Autodesk Inventor part; units mm, degrees
ref_plane "YZ Plane" through (0, 0, 0) normal (1, 0, 0) x (0, 1, 0)
ref_plane "XZ Plane" through (0, 0, 0) normal (0, 1, 0) x (-1, 0, 0)
ref_plane "XY Plane" through (0, 0, 0) normal (0, 0, 1) x (1, 0, 0)
sketch "Sketch6" plane through (0, 0, 0) normal (0, 0, 1) x (1, 0, 0)
  line L0 (20, 28) -> (24, 28)
  line L1 (24, 28) -> (24, 0)
  line L2 (24, -15) -> (20, -15)
  line L3 (20, -15) -> (20, -12)
  line L4 (17, 2) -> (20, 2)
  line L5 (20, 2) -> (20, -2) construction
  line L6 (20, -2) -> (17, -2)
  line L7 (17, -2) -> (17, 2)
  line L8 (20, -10) -> (21, -10)
  line L9 (21, -10) -> (21, -12)
  line L10 (21, -12) -> (20, -12)
  line L11 (20, -12) -> (20, -10) construction
  line L12 (20, 2) -> (20, 16)
  line L13 (20, -2) -> (20, 2) construction
  line L14 (20, -10) -> (20, -2)
  line L15 (20, -12) -> (20, -10) construction
  line L16 (0, 0) -> (0, 29.8024)
  line L17 (20, 16) -> (21, 16)
  line L18 (21, 16) -> (21, 18)
  line L19 (21, 18) -> (20, 18)
  line L20 (17, 0) -> (24, 0) construction
  line L21 (24, 0) -> (24, -15)
  line L22 (20, 18) -> (20, 28)
  line L23 (20, 16) -> (20, 18) construction
  point P0 (20, 0)
  point P1 (20, -11)
  point P2 (20.5, -10)
  dimension "d15" = 4
  dimension "d16" = 3
  dimension "d17" = 8
  dimension "d18" = 2
  dimension "d19" = 1
  dimension "d21" = 48
  dimension "d22" = 40
  dimension "d24" = 14
  dimension "d25" = 15
  dimension "d26" = 2
  dimension "d27" = 1
  dimension "d28" = 28
revolve "Revolution1" add sketch "Sketch6" angle 360 mid plane about axis through (0, 0, 0) along (0, 1, 0)
equation "\"d26\" = d18"
equation "\"d27\" = d19"
properties part number "Седло для подшипника"
Here's how the part is built. I have some questions about the finished solid (model axes, mm). A direction names the side the tool comes from. Coordinates: 2 decimals unless noted, no trailing zeros. Loops run counter-clockwise (first coordinate to the right, second up) from the corner with the lowest first, then second, coordinate; pieces in that order, holes last. Notation, with made-up numbers: (76.5, -26.75) - (104.5, -26.75) arc R11 ccw to (104.5, -21.75) - close; hole circle Ø5 at (65.5, 37.25). An arc over 180 degrees is marked (long way). Return JSON: item names as keys, results as strings. Group by question number.
Item 1: On a 3-axis mill with a long thin cutter (end or side, diameter ignored), from which of +Z, -Z, +X, -X, +Y, -Y can I reach the whole of each face in a straight line? I mean faces 4 (the face through (4.336, -5.944, -19.524)), 5 (the face through (-19, 18, -8)), 6 (the face through (4.336, 23.07, -19.524)), 7 (the face through (23.977, 6.199, -1.055)). Say none if no direction works.
Item 2: Will these pins go through, and if not, where does the flat tip stop? P1, Ø12, axis at x = -7.5, z = -15, coming from the -Y side; P2, Ø2, axis at y = 6.5, z = 7, coming from the -X side; P3, Ø1.5, axis at x = 17, y = -5, coming from the -Z side; P4, Ø1.5, axis at y = 14, z = 7.5, coming from the -X side.
Item 3: If we section it at C-C on y = 9.5: Write out the boundary of the cut face in (x, z), and give its area (3 significant figures).
Item 4: I need wall thicknesses on line 1 (Z direction, x = 0, y = 5.5); line 2 (Z direction, x = 0, y = 17.05); line 3 (Y direction, x = -8, z = -16.5). Which ranges of each line are inside material? Lowest first, please. Write a range as from..to.
Item 5: If we section it at D-D on z = 18: Write out the boundary of the cut face in (x, y).
Item 6: We'd pull the mould along Y, two halves only. Please class faces 1 (the face through (9, 2, -15)), 2 (the face through (-19, 16, -8)), 3 (the face through (5, -15, 20)): +Y half, -Y half, draft (parallel to the pull), parting line (faces both ways), or undercut.
Calculated:
{
 "1": {"face 4": "-Y", "face 5": "none", "face 6": "+Y", "face 7": "+Y, -Y"},
 "2": {"P1": "stops at y = -15", "P2": "stops at x = -23.24", "P3": "stops at z = -17.66", "P4": "stops at x = -23.03"},
 "3": {"outline": "circle Ø48 at (0, 0); hole circle Ø40 at (0, 0)", "area": "553 mm^2"},
 "4": {"line 1": "z = -24..-20, 20..24", "line 2": "z = -24..-21, 21..24", "line 3": "y = -2..2"},
 "5": {"outline": "(-15.87, -15) - (-8.72, -15) - (-8.72, -12) - (-10.82, -12) - (-10.82, -10) - (-8.72, -10) - (-8.72, -2) - (8.72, -2) - (8.72, -10) - (10.82, -10) - (10.82, -12) - (8.72, -12) - (8.72, -15) - (15.87, -15) - (15.87, 28) - (8.72, 28) - (8.72, 18) - (10.82, 18) - (10.82, 16) - (8.72, 16) - (8.72, 2) - (-8.72, 2) - (-8.72, 16) - (-10.82, 16) - (-10.82, 18) - (-8.72, 18) - (-8.72, 28) - (-15.87, 28) - close"},
 "6": {"face 1": "+Y half", "face 2": "undercut", "face 3": "-Y half"}
}
